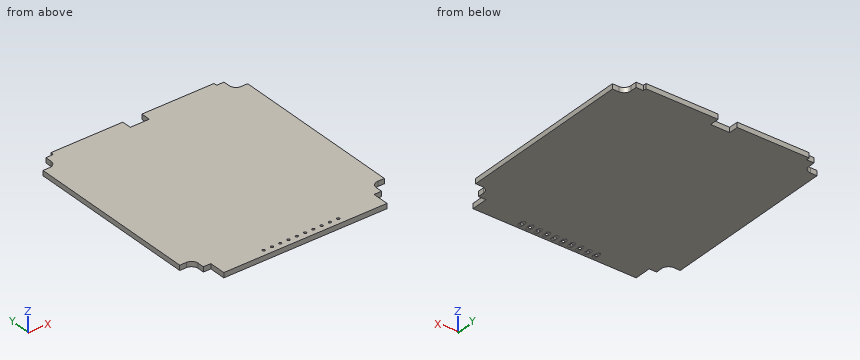
from build123d import *

# Parameters (mm, degrees)
SKETCH1_W            = 62.738
SKETCH1_H            = 67.818
PCB_DEPTH            = 1.524
CUT1_DEPTH           = 47.21857871
MIRROR3_COPY_1_DEPTH = 47.21857871
SKETCH4_W            = 5.842
SKETCH4_H            = 2.921
CUTOUT_DEPTH         = 1.524
SKETCH3_R            = 0.4064
HOLES_DEPTH          = 47.21857871
SKETCH5_R            = 0.4064
SOLDER_PAD_DEPTH     = 0.0254
LPATTERN1_COUNT      = 10
LPATTERN1_PITCH      = 2.54


with BuildPart() as part:
    # Sketch1 → PCB (new body)
    with BuildSketch(Plane.XY):
        Rectangle(SKETCH1_W, SKETCH1_H)
    extrude(amount=PCB_DEPTH)

    # Sketch2 → cut1 (cut, through all)
    with BuildSketch(Plane.XY.offset(1.524)):
        with BuildLine():
            Line((-31.369, 28.829), (-29.337, 28.829))
            ThreePointArc((-29.337, 28.829), (-27.900159021, 29.424159021), (-27.305, 30.861))
            Line((-27.305, 30.861), (-27.305, 32.893))
            Line((-27.305, 32.893), (-25.019, 32.893))
            Line((-25.019, 32.893), (-25.019, 40.259))
            Line((-25.019, 40.259), (-31.369, 40.259))
            Line((-31.369, 40.259), (-31.369, 28.829))
        make_face()
    cut1 = extrude(amount=-CUT1_DEPTH, mode=Mode.SUBTRACT)

    # Mirror1: cut1 across plane
    add(cut1.mirror(Plane(origin=(0, 0, 0), x_dir=(0, 0, 1), z_dir=(1, 0, 0))), mode=Mode.SUBTRACT)

    # Mirror3: cut1 across plane
    add(cut1.mirror(Plane(origin=(0, 2.032, 0), x_dir=(0, 0, 1), z_dir=(0, -1, 0))), mode=Mode.SUBTRACT)

    # Mirror3 copy 1 sketch → Mirror3 copy 1 (cut, through all)
    with BuildSketch(Plane(origin=(0, 4.064, 1.524), x_dir=(-1, 0, 0), z_dir=(0, 0, 1))):
        with BuildLine():
            Line((-31.369, 28.829), (-29.337, 28.829))
            ThreePointArc((-29.337, 28.829), (-27.900159021, 29.424159021), (-27.305, 30.861))
            Line((-27.305, 30.861), (-27.305, 32.893))
            Line((-27.305, 32.893), (-25.019, 32.893))
            Line((-25.019, 32.893), (-25.019, 40.259))
            Line((-25.019, 40.259), (-31.369, 40.259))
            Line((-31.369, 40.259), (-31.369, 28.829))
        make_face()
    extrude(amount=-MIRROR3_COPY_1_DEPTH, mode=Mode.SUBTRACT)

    # Sketch4 → cutout (cut)
    with BuildSketch(Plane(origin=(0, 0, 0), x_dir=(-1, 0, 0), z_dir=(0, 0, -1))):
        with Locations((0, 32.4485)):
            Rectangle(SKETCH4_W, SKETCH4_H)
    extrude(amount=-CUTOUT_DEPTH, mode=Mode.SUBTRACT)

    # Sketch3 → holes (cut, through all)
    with BuildSketch(Plane.XY.offset(1.524)):
        with Locations((-11.303, -32.004)):
            Circle(SKETCH3_R)
        with Locations((-8.763, -32.004)):
            Circle(SKETCH3_R)
        with Locations((-6.223, -32.004)):
            Circle(SKETCH3_R)
        with Locations((-3.683, -32.004)):
            Circle(SKETCH3_R)
        with Locations((-1.143, -32.004)):
            Circle(SKETCH3_R)
        with Locations((1.397, -32.004)):
            Circle(SKETCH3_R)
        with Locations((3.937, -32.004)):
            Circle(SKETCH3_R)
        with Locations((6.477, -32.004)):
            Circle(SKETCH3_R)
        with Locations((9.017, -32.004)):
            Circle(SKETCH3_R)
        with Locations((11.557, -32.004)):
            Circle(SKETCH3_R)
    extrude(amount=-HOLES_DEPTH, mode=Mode.SUBTRACT)

    # Sketch5 → solder pad (add)
    with BuildSketch(Plane(origin=(0, 0, 0), x_dir=(-1, 0, 0), z_dir=(0, 0, -1))):
        with BuildLine():
            Line((-12.192, -31.369), (-12.192, -32.639))
            ThreePointArc((-12.192, -32.639), (-11.557, -33.274), (-10.922, -32.639))
            Line((-10.922, -32.639), (-10.922, -31.369))
            ThreePointArc((-10.922, -31.369), (-11.557, -30.734), (-12.192, -31.369))
        make_face()
        with Locations(Location((-11.557, -32.004, 0), (0, 0, 180))):
            Circle(SKETCH5_R, mode=Mode.SUBTRACT)
    solder_pad = extrude(amount=SOLDER_PAD_DEPTH)

    # LPattern1: solder pad ×10
    with Locations(*[(-i * LPATTERN1_PITCH, 0, 0) for i in range(1, LPATTERN1_COUNT)]):
        add(solder_pad)


solid = part.part
Geometry check sheet. Reference: the model listing, model coordinates, mm. Round coordinates to 2 decimals unless told otherwise and drop trailing zeros. Loops run counter-clockwise (first coordinate to the right, second up) from the corner with the lowest first, then second, coordinate; pieces in that order, holes last. Notation, with made-up numbers: (25, 83.5) - (75, 83.5) arc R14 ccw to (75, 89.5) - close; hole circle Ø11 at (71, 54.25). An arc over 180 degrees is marked (long way). Answer as CSV lines item,"result".
(1) Cross-section at B-B, the plane x = 16.5. Enter the section's corners in (y, z).
Output values:
outline,"(-33.91, 0) - (33.91, 0) - (33.91, 1.52) - (-33.91, 1.52) - close"
(2) Depth check by flat-ended pin: pin 1 Ø0.8 at (x, z) = (-26.5, 1) entering from +Y; pin 2 Ø0.5 at (x, z) = (-1.5, 0.5) entering from +Y; pin 3 Ø0.8 at (y, z) = (-27.5, 0.5) entering from -X (3 decimals). Enter the tip coordinate at first touch or a pass-through.
Output values:
pin 1,"stops at y = 32.89"
pin 2,"stops at y = 30.99"
pin 3,"stops at x = -27.305"
(3) Cross-section at C-C, the plane z = 0.55. Give the number of separate pieces and of enclosed holes in the cut face, and give its area (3 significant figures).
Output values:
separate pieces,"1"
enclosed holes,"10"
area,"4,090 mm²"
(4) Cross-section at A-A, the plane y = -23.5. Enter the section's corners in (x, z), and give its area (3 significant figures).
Output values:
outline,"(-31.37, 0) - (31.37, 0) - (31.37, 1.52) - (-31.37, 1.52) - close"
area,"95.6 mm²"
(5) Material ranges on line 1 along X through (y, z) = (-31, 1.35); line 2 along Z through (x, y) = (-22, 26); line 3 along Y through (x, z) = (-25.5, 1.1), recorded low to high.
Output values:
line 1,"x = -25.02 to 25.02"
line 2,"z = 0 to 1.52"
line 3,"y = -28.83 to 32.89"
